from build123d import *

# Parameters (mm, degrees)
SKETCH_W        = 63
SKETCH_H        = 75
PAD_DEPTH       = 12
PAD001_DEPTH    = 63
SKETCH002_W     = 19
SKETCH002_H     = 22.106678
POCKET_DEPTH    = 75.001
SKETCH003_W     = 25
SKETCH003_H     = 65.320022
POCKET001_DEPTH = 15
SKETCH004_W     = 25
SKETCH004_H     = 5
PAD002_DEPTH    = 1
PAD003_DEPTH    = 25


with BuildPart() as part:
    # Sketch → Pad (new body)
    with BuildSketch(Plane.XY):
        Rectangle(SKETCH_W, SKETCH_H)
    extrude(amount=PAD_DEPTH)

    # Sketch001 → Pad001 (new body)
    with BuildSketch(Plane.YZ.offset(31.5)):
        Polygon((-37.260017, 12), (37.5, 50), (37.5, 12), align=None)
    extrude(amount=-PAD001_DEPTH)

    # Sketch002 → Pocket (cut, through all)
    with BuildSketch(Plane(origin=(0, 37.5, 0), x_dir=(-1, 0, 0), z_dir=(0, 1, 0))):
        with Locations((0, 49.053339)):
            Rectangle(SKETCH002_W, SKETCH002_H)
    extrude(amount=-POCKET_DEPTH, mode=Mode.SUBTRACT)

    # Sketch003 → Pocket001 (cut)
    with BuildSketch(Plane.YZ.offset(31.5)):
        with Locations((0, 22.23333)):
            Rectangle(SKETCH003_W, SKETCH003_H)
    extrude(amount=-POCKET001_DEPTH, mode=Mode.SUBTRACT)

    # Sketch004 → Pad002 (new body)
    with BuildSketch(Plane(origin=(0, -12.497267, 24.586735), x_dir=(1, 0, 0), z_dir=(0, -0.453118, 0.89145))):
        with Locations((0, -5.278043)):
            Rectangle(SKETCH004_W, SKETCH004_H)
    extrude(amount=PAD002_DEPTH)

    # Sketch005 → Pad003 (new body)
    with BuildSketch(Plane(origin=(-12.5, 0, 0), x_dir=(0, -1, 0), z_dir=(-1, 0, 0))):
        Polygon((-4.915291, 33.437417), (26.562611, 17.437417), (26.562611, 33.437417), align=None)
    extrude(amount=-PAD003_DEPTH)


solid = part.part
Geometry: final body of the model. Coordinates: model frame, mm. A direction names the side the tool comes from. Coordinates: 2 decimals unless noted, no trailing zeros. Order: outer loops, then holes, each group sorted by start corner. A loop starts at its lowest first (then second) coordinate and runs counter-clockwise, first axis right, second up.
(1) Section query D-D (z = 4.5). Return the cut outline in (x, y).
(2) Draft query along X for faces 4 (the face through (0, -37.5, 6)), 5 (the face through (-9.5, 28, 43)), 6 (the face through (-31.5, 9, 20)), 7 (the face through (31.5, 25, 20)). Return one class per face: pulls with the +X half, pulls with the -X half, needs draft (parallel to the pull), parting line crosses it, or undercut.
(3) Section query A-A (x = 25). Return the cut outline in (y, z).
(4) Section query B-B (z = 39.5). Return the cut outline in (x, y).
(5) Material intervals for probe 1 along Y at (x, z) = (19, 6.5); probe 2 along X at (y, z) = (-5, 7); probe 3 along Y at (x, z) = (1, 20.5), sorted ascending.
(6) First-contact query: pin 1 (17.5 mm diameter, centred on x = -4, z = 21.5, fed in from -Y); pin 2 (3 mm diameter, centred on x = -5.5, y = 29.5, fed in from +Z); pin 3 (3 mm diameter, centred on x = 20.5, z = 23.5, fed in from -Y). Flat tips, straight axial feed; report the tip coordinate or a pass-through.
(7) Section query C-C (x = 5.5). Return the cut outline in (y, z), plus the area to 3 significant figures.
(8) Access query for faces 1 (the face through (-12.5, -16, 27)), 2 (the face through (12.5, -18, 29)), 3 (the face through (0, 26, 38)). Directions: +Z, -Z, +X, -X, +Y, -Y. A direction counts if a zero-diameter tool reaches every point of the face in a straight line with its end or side. Return the directions, or none.
Solution:
1. outline: (-31.5, -37.5) - (31.5, -37.5) - (31.5, -12.5) - (16.5, -12.5) - (16.5, 12.5) - (31.5, 12.5) - (31.5, 37.5) - (-31.5, 37.5) - close
2. face 4: needs draft
2. face 5: undercut
2. face 6: pulls with the -X half
2. face 7: pulls with the +X half
3. outline: (-37.5, 0) - (-12.5, 0) - (-12.5, 24.59) - (-37.26, 12) - (-37.5, 12) - close; (12.5, 0) - (37.5, 0) - (37.5, 50) - (12.5, 37.29) - close
4. outline: (-31.5, 16.84) - (-9.5, 16.84) - (-9.5, 37.5) - (-31.5, 37.5) - close; (9.5, 16.84) - (31.5, 16.84) - (31.5, 37.5) - (9.5, 37.5) - close
5. probe 1: y = -37.5 to -12.5, 12.5 to 37.5
5. probe 2: x = -31.5 to 16.5
5. probe 3: y = -26.56 to 37.5
6. pin 1: stops at y = -35.78
6. pin 2: stops at z = 38
6. pin 3: stops at y = -17.59
7. outline: (-37.5, 0) - (37.5, 0) - (37.5, 38) - (13.89, 38) - (4.92, 33.44) - (-26.56, 33.44) - (-26.56, 17.44) - (-37.26, 12) - (-37.5, 12) - close
7. area: 2,430 mm2
8. face 1: +Z, -X, -Y
8. face 2: +Z, +X, -Y
8. face 3: +Z, +Y, -Y
